Job drawing, mm, ordinate dimensions from the low corner. One solid piece. A direction names the side the tool comes from. Give positions to 0.01 mm unless a question says otherwise; leave off trailing zeros. Loops run counter-clockwise (first coordinate to the right, second up) from the corner with the lowest first, then second, coordinate; pieces in that order, holes last. Notation, with made-up numbers: (75.25, 47) -> (132.25, 47) arc R31 cw to (132.25, 73) -> close; hole circle Ø10 at (87.25, 80.25). An arc over 180 degrees is marked (long way). Answer as a JSON object with one key per item and string values. Group by question number.
Q1. Tool access for the marked faces 4 and 5: list every direction of +Z, -Z, +X, -X, +Y, -Y with a clear straight run to the whole face (end or side of a thin tool).
Q2. Two-plate mould, pull along X, no slides. Class the marked faces 1, 2 and 3: pulls with the +X half, pulls with the -X half, needs draft (parallel to the pull), parting line crosses it, or undercut.
Q3. Band-saw the part on C-C, the plane x = 35. Write the cut outline in (y, z) (3 decimals), plus the area to 3 significant figures.
Q4. Wall check: probe 1 along X at (y, z) = (14, 174) (3 decimals); probe 2 along Z at (x, y) = (37, 17.5) (3 decimals); probe 3 along Y at (x, z) = (27.5, 190.5) (3 decimals). Give the ranges that are in metal, low to high. Write a range as from..to.
Q5. Drop a flat-ended pin along its axis: pin 1 (5 mm diameter, centred on x = 20, z = 77, fed in from +Y) (3 decimals). Give the stop position or say it passes through.
Q6. Band-saw the part on B-B, the plane z = 190. Write the cut outline in (x, y) (3 decimals).
Q7. Band-saw the part on A-A, the plane y = 11. Write the cut outline in (x, z) (3 decimals).
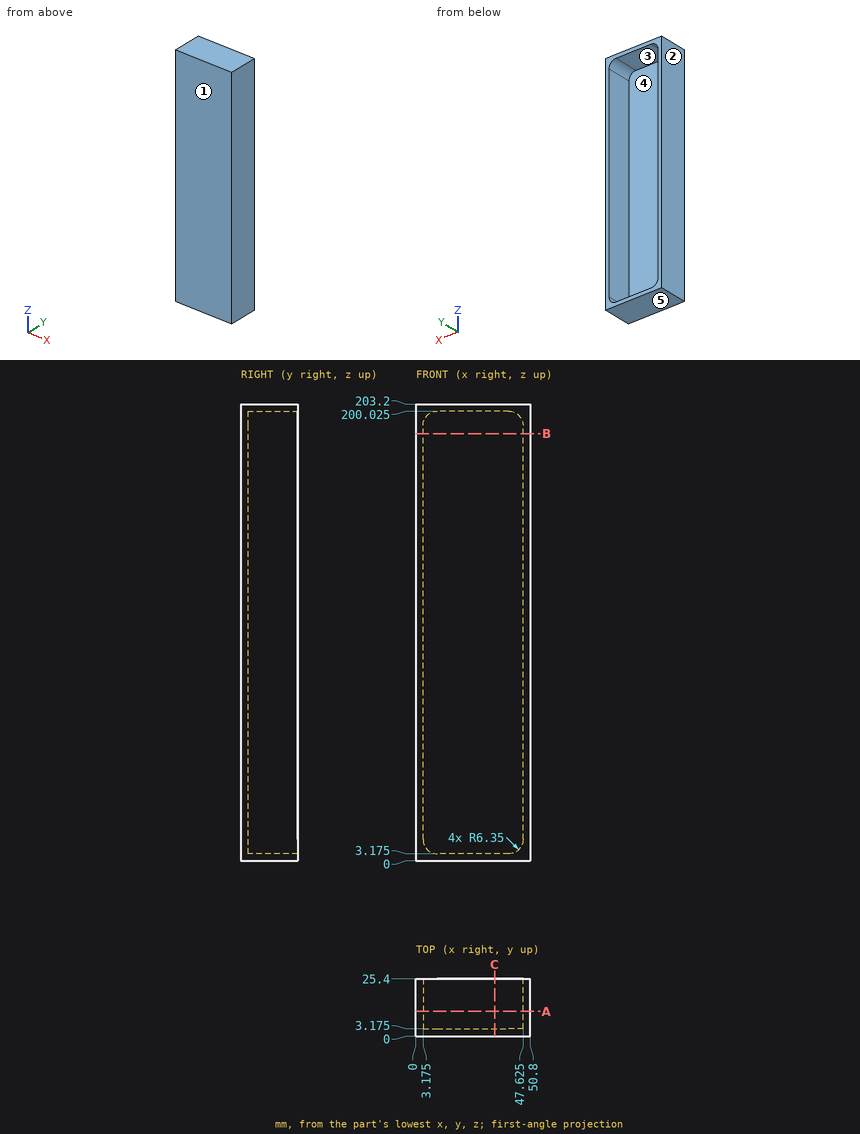
Worked answers:
{
 "1": {"face 4": "+Y", "face 5": "-Z, +X, -X, +Y, -Y"},
 "2": {"face 1": "needs draft", "face 2": "pulls with the -X half", "face 3": "undercut"},
 "3": {"outline": "(0, 0) -> (25.4, 0) -> (25.4, 3.175) -> (3.175, 3.175) -> (3.175, 200.025) -> (25.4, 200.025) -> (25.4, 203.2) -> (0, 203.2) -> close", "area": "786 mm2"},
 "4": {"probe 1": "0..3.175, 47.625..50.8", "probe 2": "0..3.175, 200.025..203.2", "probe 3": "0..3.175"},
 "5": {"pin 1": "y = 3.175"},
 "6": {"outline": "(0, 0) -> (50.8, 0) -> (50.8, 25.4) -> (47.625, 25.4) -> (47.625, 3.175) -> (3.175, 3.175) -> (3.175, 25.4) -> (0, 25.4) -> close"},
 "7": {"outline": "(0, 0) -> (50.8, 0) -> (50.8, 203.2) -> (0, 203.2) -> close; hole (3.175, 9.525) arc R6.35 ccw to (9.525, 3.175) -> (41.275, 3.175) arc R6.35 ccw to (47.625, 9.525) -> (47.625, 193.675) arc R6.35 ccw to (41.275, 200.025) -> (9.525, 200.025) arc R6.35 ccw to (3.175, 193.675) -> close"}
}
